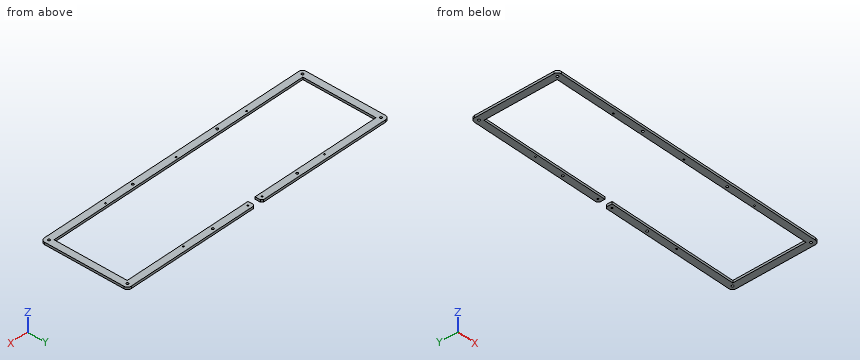
```python
from build123d import *

# Parameters (mm, degrees)
MODEL_R             = 1.45
MODEL_R_2           = 0.95
BOSS_EXTRUDE1_DEPTH = 3


with BuildPart() as part:
    # Model → Boss-Extrude1 (new body)
    with BuildSketch(Plane.XY):
        with BuildLine():
            Line((5, 113.6), (178.3875, 113.6))
            Line((178.3875, 113.6), (180.3875, 111.6))
            Line((180.3875, 111.6), (180.3875, 104.6))
            Line((180.3875, 104.6), (9, 104.6))
            Line((9, 104.6), (9, 9))
            Line((9, 9), (361.775, 9))
            Line((361.775, 9), (361.775, 104.6))
            Line((361.775, 104.6), (190.3875, 104.6))
            Line((190.3875, 104.6), (190.3875, 111.6))
            Line((190.3875, 111.6), (192.3875, 113.6))
            Line((192.3875, 113.6), (365.775, 113.6))
            ThreePointArc((365.775, 113.6), (369.310533906, 112.135533906), (370.775, 108.6))
            Line((370.775, 108.6), (370.775, 5))
            ThreePointArc((370.775, 5), (369.310533906, 1.464466094), (365.775, 0))
            Line((365.775, 0), (5, 0))
            ThreePointArc((5, 0), (1.464466094, 1.464466094), (0, 5))
            Line((0, 5), (0, 108.6))
            ThreePointArc((0, 108.6), (1.464466094, 112.135533906), (5, 113.6))
        make_face()
        with Locations((245.275, 109.1)):
            Circle(MODEL_R, mode=Mode.SUBTRACT)
        with Locations((125.5, 109.1)):
            Circle(MODEL_R, mode=Mode.SUBTRACT)
        with Locations((245.275, 4.5)):
            Circle(MODEL_R, mode=Mode.SUBTRACT)
        with Locations((285.3875, 6)):
            Circle(MODEL_R_2, mode=Mode.SUBTRACT)
        with Locations((185.3875, 6)):
            Circle(MODEL_R_2, mode=Mode.SUBTRACT)
        with Locations((85.3875, 6)):
            Circle(MODEL_R_2, mode=Mode.SUBTRACT)
        with Locations((285.3875, 107.6)):
            Circle(MODEL_R_2, mode=Mode.SUBTRACT)
        with Locations((85.3875, 107.6)):
            Circle(MODEL_R_2, mode=Mode.SUBTRACT)
        with Locations((365.275, 108.1)):
            Circle(MODEL_R, mode=Mode.SUBTRACT)
        with Locations((365.275, 5.5)):
            Circle(MODEL_R, mode=Mode.SUBTRACT)
        with Locations((5.5, 5.5)):
            Circle(MODEL_R, mode=Mode.SUBTRACT)
        with Locations((5.5, 108.1)):
            Circle(MODEL_R, mode=Mode.SUBTRACT)
        with Locations((175.3875, 109.1)):
            Circle(MODEL_R_2, mode=Mode.SUBTRACT)
        with Locations((195.3875, 109.1)):
            Circle(MODEL_R_2, mode=Mode.SUBTRACT)
        with Locations((125.5, 4.5)):
            Circle(MODEL_R, mode=Mode.SUBTRACT)
    extrude(amount=BOSS_EXTRUDE1_DEPTH)


solid = part.part
```
Part model, mm, in its own coordinate system. Round coordinates to 2 decimals unless told otherwise and drop trailing zeros. Loops run counter-clockwise (first coordinate to the right, second up) from the corner with the lowest first, then second, coordinate; pieces in that order, holes last.
Item 1: Drop a flat-ended pin along its axis: P1, Ø1.7, axis at x = 245.275, y = 109.1, coming from the -Z side. Give the stop position or say it passes through.
Item 2: Cut at B-B, the plane y = 81. Give the cut face in (x, z) (3 decimals).
Item 3: Cut at A-A, the plane x = 94. Give the cut face in (y, z), then the cut area to 3 significant figures.
Item 4: Cut at C-C, the plane z = 1.25. State how many separate pieces and enclosed holes the cut face has, then the cut area to 3 significant figures.
Item 5: Drill centre lines: line 1 (Y direction, x = 125.5, z = 1.5); line 2 (Y direction, x = 54, z = 1.7); line 3 (X direction, y = 34.5, z = 2.5) (3 decimals). Where is each one in solid material? Low to high.
A:
1. P1: passes through
2. outline: (0, 0) - (9, 0) - (9, 3) - (0, 3) - close; (361.775, 0) - (370.775, 0) - (370.775, 3) - (361.775, 3) - close
3. outline: (0, 0) - (9, 0) - (9, 3) - (0, 3) - close; (104.6, 0) - (113.6, 0) - (113.6, 3) - (104.6, 3) - close
3. area: 54.0 mm2
4. separate pieces: 1
4. enclosed holes: 15
4. area: 8,210 mm2
5. line 1: y = 0 to 3.05, 5.95 to 9, 104.6 to 107.65, 110.55 to 113.6
5. line 2: y = 0 to 9, 104.6 to 113.6
5. line 3: x = 0 to 9, 361.775 to 370.775
